from build123d import *

# Parameters (mm, degrees)
SKETCH_1_R          = 1.5
SKETCH_1_R_2        = 22.5
EXTRUDE_1_DEPTH     = 3
SKETCH_2_R          = 2
SKETCH_2_R_2        = 1.75
CUT_EXTRUDE_1_DEPTH = 10
SKETCH_3_R          = 1.5
SKETCH_3_R_2        = 1.75
SKETCH_3_R_3        = 22.5
CUT_EXTRUDE_2_DEPTH = 10
SKETCH_4_R          = 1.5
CUT_EXTRUDE_3_DEPTH = 10
SKETCH_5_R          = 1.5
CUT_EXTRUDE_4_DEPTH = 95.387499172


with BuildPart() as part:
    # 草图1 → 凸台-拉伸1 (new body)
    with BuildSketch(Plane.XY):
        with BuildLine():
            Line((-10, 50), (-350, 50))
            ThreePointArc((-350, 50), (-400, 0), (-350, -50))
            Line((-350, -50), (-10, -50))
            ThreePointArc((-10, -50), (40, 0), (-10, 50))
        make_face()
        with Locations((-387.5, 0)):
            Circle(SKETCH_1_R, mode=Mode.SUBTRACT)
        with Locations((-378.726666617, 24.104535363)):
            Circle(SKETCH_1_R, mode=Mode.SUBTRACT)
        with Locations((-356.511806663, 36.930290738)):
            Circle(SKETCH_1_R, mode=Mode.SUBTRACT)
        with Locations((-331.25, 32.475952642)):
            Circle(SKETCH_1_R, mode=Mode.SUBTRACT)
        with Locations((-314.761526721, 12.825755375)):
            Circle(SKETCH_1_R, mode=Mode.SUBTRACT)
        with Locations((-314.761526721, -12.825755375)):
            Circle(SKETCH_1_R, mode=Mode.SUBTRACT)
        with Locations((-331.25, -32.475952642)):
            Circle(SKETCH_1_R, mode=Mode.SUBTRACT)
        with Locations((-356.511806663, -36.930290738)):
            Circle(SKETCH_1_R, mode=Mode.SUBTRACT)
        with Locations((-378.726666617, -24.104535363)):
            Circle(SKETCH_1_R, mode=Mode.SUBTRACT)
        with Locations((-350, 0)):
            Circle(SKETCH_1_R_2, mode=Mode.SUBTRACT)
        with Locations((-10, 0)):
            Circle(SKETCH_1_R_2, mode=Mode.SUBTRACT)
        with Locations((18.726666617, -24.104535363)):
            Circle(SKETCH_1_R, mode=Mode.SUBTRACT)
        with Locations((-3.488193337, -36.930290738)):
            Circle(SKETCH_1_R, mode=Mode.SUBTRACT)
        with Locations((-28.75, -32.475952642)):
            Circle(SKETCH_1_R, mode=Mode.SUBTRACT)
        with Locations((-45.238473279, -12.825755375)):
            Circle(SKETCH_1_R, mode=Mode.SUBTRACT)
        with Locations((-45.238473279, 12.825755375)):
            Circle(SKETCH_1_R, mode=Mode.SUBTRACT)
        with Locations((-28.75, 32.475952642)):
            Circle(SKETCH_1_R, mode=Mode.SUBTRACT)
        with Locations((-3.488193337, 36.930290738)):
            Circle(SKETCH_1_R, mode=Mode.SUBTRACT)
        with Locations((18.726666617, 24.104535363)):
            Circle(SKETCH_1_R, mode=Mode.SUBTRACT)
        with Locations((27.5, 0)):
            Circle(SKETCH_1_R, mode=Mode.SUBTRACT)
    extrude(amount=EXTRUDE_1_DEPTH)

    # 草图2 → 切除-拉伸1 (cut)
    with BuildSketch(Plane(origin=(0, 0, 0), x_dir=(-1, 0, 0), z_dir=(0, 0, -1))):
        with Locations((39, 0)):
            Circle(SKETCH_2_R)
        with Locations(Location((321, 0, 0), (0, 0, 180))):
            Circle(SKETCH_2_R_2)
    extrude(amount=-CUT_EXTRUDE_1_DEPTH, mode=Mode.SUBTRACT)

    # 草图3 → 切除-拉伸2 (cut)
    with BuildSketch(Plane(origin=(0, 0, 0), x_dir=(-1, 0, 0), z_dir=(0, 0, -1))):
        with BuildLine():
            Line((80, -50), (180, -50))
            Line((180, -50), (350, -50))
            ThreePointArc((350, -50), (400, 0), (350, 50))
            Line((350, 50), (80, 50))
            Line((80, 50), (80, -50))
        make_face()
        with Locations((331.25, -32.475952642)):
            Circle(SKETCH_3_R, mode=Mode.SUBTRACT)
        with Locations((356.511806663, -36.930290738)):
            Circle(SKETCH_3_R, mode=Mode.SUBTRACT)
        with Locations((378.726666617, -24.104535363)):
            Circle(SKETCH_3_R, mode=Mode.SUBTRACT)
        with Locations((314.761526721, -12.825755375)):
            Circle(SKETCH_3_R, mode=Mode.SUBTRACT)
        with Locations((321, 0)):
            Circle(SKETCH_3_R_2, mode=Mode.SUBTRACT)
        with Locations((314.761526721, 12.825755375)):
            Circle(SKETCH_3_R, mode=Mode.SUBTRACT)
        with Locations((350, 0)):
            Circle(SKETCH_3_R_3, mode=Mode.SUBTRACT)
        with Locations((387.5, 0)):
            Circle(SKETCH_3_R, mode=Mode.SUBTRACT)
        with Locations((331.25, 32.475952642)):
            Circle(SKETCH_3_R, mode=Mode.SUBTRACT)
        with Locations((378.726666617, 24.104535363)):
            Circle(SKETCH_3_R, mode=Mode.SUBTRACT)
        with Locations((356.511806663, 36.930290738)):
            Circle(SKETCH_3_R, mode=Mode.SUBTRACT)
    extrude(amount=-CUT_EXTRUDE_2_DEPTH, mode=Mode.SUBTRACT)

    # 草图4 → 切除-拉伸3 (cut)
    with BuildSketch(Plane(origin=(0, 0, 0), x_dir=(-1, 0, 0), z_dir=(0, 0, -1))):
        with Locations((-36.25, 0)):
            Circle(SKETCH_4_R)
        with Locations((-13.125, 40.053674925)):
            Circle(SKETCH_4_R)
        with Locations((33.125, 40.053674925)):
            Circle(SKETCH_4_R)
        with Locations((56.25, 0)):
            Circle(SKETCH_4_R)
        with Locations((33.125, -40.053674925)):
            Circle(SKETCH_4_R)
        with Locations((-13.125, -40.053674925)):
            Circle(SKETCH_4_R)
    extrude(amount=-CUT_EXTRUDE_3_DEPTH, mode=Mode.SUBTRACT)

    # 草图5 → 切除-拉伸4 (cut, through all)
    with BuildSketch(Plane.XY.offset(3)):
        with Locations((-70, 40.051993223)):
            Circle(SKETCH_5_R)
        with Locations((-50, 40.051993223)):
            Circle(SKETCH_5_R)
        with Locations((-70.013968461, -40.048849195)):
            Circle(SKETCH_5_R)
        with Locations((-50, -40.048849193)):
            Circle(SKETCH_5_R)
    extrude(amount=-CUT_EXTRUDE_4_DEPTH, mode=Mode.SUBTRACT)


solid = part.part
Check sheet for the modelled part. Datum: model origin and axes. Units: mm. Give positions to 0.01 mm unless a question says otherwise; leave off trailing zeros. Loops run counter-clockwise (first coordinate to the right, second up) from the corner with the lowest first, then second, coordinate; pieces in that order, holes last. Notation, with made-up numbers: M 58.25,-24 L 114.25,-24 A29 ccw 114.25,1 Z; hole C 20.25,-16 d9. An arc over 180 degrees is marked long. Use a Markdown table: item, result. Add a question column.
Q1. Mould release check, pull along X, two halves, no side actions. Record for faces 1 (the flat face through (-45, 50, 1)), 2 (the flat face through (-80, 1, 1)), 3 (the cylindrical face through (0.382, -19.961, 1.479)): pulls with the +X half, pulls with the -X half, needs draft (parallel to the pull), parting line crosses it, or undercut.
Q2. Scan lines: line 1 along Y through (x, z) = (-69, 2.7); line 2 along Y through (x, z) = (-56.25, 2.1); line 3 along Y through (x, z) = (-28.75, 0.9). Record each from-to range of solid material in increasing order. Write a range as [from, to].
Q3. Sectioned sample at C-C, the plane x = -70. Record the cut outline in (y, z).
Q4. Sectioned sample at B-B, the plane y = -6. Record the cut outline in (x, z), then the cut area to 3 significant figures.
Q5. Sectioned sample at A-A, the plane x = -39. Record the cut outline in (y, z).
Q6. Sectioned sample at D-D, the plane z = 2.45. Give the number of separate pieces and of enclosed holes in the cut face, then the cut area to 3 significant figures.
Verdict:
| question | item | result |
|---|---|---|
| 1 | face 1 | needs draft |
| 1 | face 2 | pulls with the -X half |
| 1 | face 3 | undercut |
| 2 | line 1 | [-50, -41.15], [-38.94, 38.93], [41.17, 50] |
| 2 | line 2 | [-50, -1.5], [1.5, 50] |
| 2 | line 3 | [-50, -33.98], [-30.98, -12.44], [12.44, 30.98], [33.98, 50] |
| 3 | outline | M -50,0 L -41.55,0 L -41.55,3 L -50,3 Z; M -38.55,0 L 38.55,0 L 38.55,3 L -38.55,3 Z; M 41.55,0 L 50,0 L 50,3 L 41.55,3 Z |
| 4 | outline | M -80,0 L -31.69,0 L -31.69,3 L -80,3 Z; M 11.69,0 L 39.64,0 L 39.64,3 L 11.69,3 Z |
| 4 | area | 229 mm^2 |
| 5 | outline | M -50,0 L -2,0 L -2,3 L -50,3 Z; M 2,0 L 50,0 L 50,3 L 2,3 Z |
| 6 | separate pieces | 1 |
| 6 | enclosed holes | 21 |
| 6 | area | 9,190 mm^2 |
